from build123d import *

# Parameters (mm, degrees)
F0_R     = 11.125
F1_DEPTH = 7


with BuildPart() as f1:
    # F0 (on Top) → F1 (new body)
    with BuildSketch(Plane.XY):
        with BuildLine():
            Line((7.176464, 36.03), (-7.176464, 36.03))
            Line((-7.176464, 36.03), (-14.352928, 23.6))
            Line((-14.352928, 23.6), (-9.68437, 15.51382))
            ThreePointArc((-9.68437, 15.51382), (-9.046046, 12.45302), (-10.350576, 9.611514))
            ThreePointArc((-10.350576, 9.611514), (-12.232609, 7.0625), (-13.499103, 4.158105))
            ThreePointArc((-13.499103, 4.158105), (-15.307655, 1.607595), (-18.277547, 0.63))
            Line((-18.277547, 0.63), (-27.614663, 0.63))
            Line((-27.614663, 0.63), (-34.791127, -11.8))
            Line((-34.791127, -11.8), (-27.614663, -24.23))
            Line((-27.614663, -24.23), (-13.261736, -24.23))
            Line((-13.261736, -24.23), (-8.593178, -16.14382))
            ThreePointArc((-8.593178, -16.14382), (-6.261609, -14.060615), (-3.148527, -13.769619))
            ThreePointArc((-3.148527, -13.769619), (0, -14.125), (3.148527, -13.769619))
            ThreePointArc((3.148527, -13.769619), (6.261609, -14.060615), (8.593178, -16.14382))
            Line((8.593178, -16.14382), (13.261736, -24.23))
            Line((13.261736, -24.23), (27.614663, -24.23))
            Line((27.614663, -24.23), (34.791127, -11.8))
            Line((34.791127, -11.8), (27.614663, 0.63))
            Line((27.614663, 0.63), (18.277547, 0.63))
            ThreePointArc((18.277547, 0.63), (15.307655, 1.607595), (13.499103, 4.158105))
            ThreePointArc((13.499103, 4.158105), (12.232609, 7.0625), (10.350576, 9.611514))
            ThreePointArc((10.350576, 9.611514), (9.046046, 12.45302), (9.68437, 15.51382))
            Line((9.68437, 15.51382), (14.352928, 23.6))
            Line((14.352928, 23.6), (7.176464, 36.03))
        make_face()
        Polygon((-31.327026, -11.8), (-25.882613, -2.37), (-14.993786, -2.37), (-9.549373, -11.8), (-14.993786, -21.23), (-25.882613, -21.23), align=None, mode=Mode.SUBTRACT)
        Polygon((25.882613, -21.23), (14.993786, -21.23), (9.549373, -11.8), (14.993786, -2.37), (25.882613, -2.37), (31.327026, -11.8), align=None, mode=Mode.SUBTRACT)
        Circle(F0_R, mode=Mode.SUBTRACT)
        Polygon((-10.888826, 23.6), (-5.444413, 33.03), (5.444413, 33.03), (10.888826, 23.6), (5.444413, 14.17), (-5.444413, 14.17), align=None, mode=Mode.SUBTRACT)
    extrude(amount=F1_DEPTH)


solid = f1.part
CAD build for the part. Positions are in the model's coordinates, mm. A direction names the side the tool comes from. Give positions to 0.01 mm unless a question says otherwise; leave off trailing zeros. Loops run counter-clockwise (first coordinate to the right, second up) from the corner with the lowest first, then second, coordinate; pieces in that order, holes last. Notation, with made-up numbers: M 5,35 L 41,35 A14 ccw 41,45 Z; hole C -15.5,65 d11. An arc over 180 degrees is marked long. One line per question, with ' | ' between items. Start each with the question number.
1. Saw through at B-B on x = 21. Give the cut face in (y, z), plus the area to 3 significant figures.
2. 3-axis set-ups, long thin cutter, end or side, ignore diameter. For faces 4 (the face through (-10.96, -20.24, 3.45)), 5 (the face through (-21, -2.37, 3)), 6 (the face through (11.986, 19.5, 3.451)): which of +Z, -Z, +X, -X, +Y, -Y reach the whole face in a straight line?
3. Flat gauge pins, fed straight in: pin 1 (2 mm diameter, centred on y = -15, z = 2.5, fed in from -X); pin 2 (3 mm diameter, centred on y = 15.5, z = 6, fed in from +X); pin 3 (2 mm diameter, centred on x = -2, z = 2.5, fed in from -Y). Where does each tip first touch, or does it go through?
4. Saw through at D-D on z = 2.25. State how many separate pieces and enclosed holes the cut face has, plus the area to 3 significant figures.
5. Probe L1, parallel to Y at x = 0, z = 3 (3 decimals); L2, parallel to X at y = -13, z = 1.5; L3, parallel to Y at x = 23.5, z = 3.5. List the from-to ranges inside material, lowest first. Write a range as from..to.
6. Saw through at A-A on x = 0. Give the cut face in (y, z) (3 decimals).
7. Two-plate mould, pull along X, no slides. Class faces 1 (the face through (-21, -24.23, 3)), 2 (the face through (-12.05, 19.61, 3.45)), 3 (the face through (-28.567, -16.581, 3.451)): pulls with the +X half, pulls with the -X half, needs draft (parallel to the pull), parting line crosses it, or undercut.
8. Saw through at C-C on y = -7. Give the cut face in (x, z), plus the area to 3 significant figures.
Result sheet:
1) outline: M -24.23,0 L -21.23,0 L -21.23,7 L -24.23,7 Z; M -2.37,0 L 0.63,0 L 0.63,7 L -2.37,7 Z | area: 42.0 mm^2
2) face 4: +Z, -Z, -Y | face 5: +Z, -Z | face 6: +Z, -Z, +X
3) pin 1: stops at x = -33.52 | pin 2: stops at x = 10.54 | pin 3: stops at y = -14.09
4) separate pieces: 1 | enclosed holes: 4 | area: 837 mm^2
5) L1: y = -14.125..-11.125, 11.125..14.17, 33.03..36.03 | L2: x = -34.1..-30.63, -10.24..10.24, 30.63..34.1 | L3: y = -24.23..-21.23, -2.37..0.63
6) outline: M -14.125,0 L -11.125,0 L -11.125,7 L -14.125,7 Z; M 11.125,0 L 14.17,0 L 14.17,7 L 11.125,7 Z; M 33.03,0 L 36.03,0 L 36.03,7 L 33.03,7 Z
7) face 1: needs draft | face 2: pulls with the -X half | face 3: undercut
8) outline: M -32.02,0 L -28.56,0 L -28.56,7 L -32.02,7 Z; M -12.32,0 L -8.65,0 L -8.65,7 L -12.32,7 Z; M 8.65,0 L 12.32,0 L 12.32,7 L 8.65,7 Z; M 28.56,0 L 32.02,0 L 32.02,7 L 28.56,7 Z | area: 99.9 mm^2
